Here's how the part is built. I have some questions about the finished solid (model axes, mm). A direction names the side the tool comes from. Coordinates: 2 decimals unless noted, no trailing zeros. Order: outer loops, then holes, each group sorted by start corner. A loop starts at its lowest first (then second) coordinate and runs counter-clockwise, first axis right, second up. Notation, with made-up numbers: (-8, -31) - (6, -31) arc R24 cw to (6, -5) - close; hole circle Ø4 at (-28, 10.5). An arc over 180 degrees is marked (long way). Answer in a Markdown table with one row per item. Add a question column.
Item 1: I want a section at A-A (z = 6). Please give me the cut outline in (x, y).
Item 2: On a 3-axis mill with a long thin cutter (end or side, diameter ignored), from which of +Z, -Z, +X, -X, +Y, -Y can I reach the whole of each face in a straight line? I mean faces 1 (the flat face through (44.45, 23, 27)), 2 (the cylindrical face through (15.755, -35.203, 37.922)), 3 (the flat face through (5.08, 32, 39)), 4 (the flat face through (7, -25.4, 7)). Say none if no direction works.
Item 3: I want a section at B-B (x = 9.5). Please give me the cut outline in (y, z).
Item 4: Will these pins go through, and if not, where does the flat tip stop? pin 1 Ø4.5 at (y, z) = (31.5, 42) entering from -X; pin 2 Ø8 at (x, y) = (21, -28.5) entering from +Z.
Item 5: If I drill on line 1 along Y through (x, z) = (37, 39.5); line 2 along Y through (x, z) = (29.5, 45.5); line 3 along Y through (x, z) = (5, 4), over which ranges is the centre line in solid material (lowest first)? Write a range as from..to.
Item 6: I want a section at D-D (z = 44). Please give me the cut outline in (x, y), plus the area to 3 significant figures.
Item 7: I want a section at C-C (y = -2). Please give me the cut outline in (x, z).
```python
from build123d import *

# Parameters (mm, degrees)
F0_W      = 50.8
F0_H      = 50.8
F1_DEPTH  = 50.8
F2_W      = 25.4
F2_H      = 25.4
F3_DEPTH  = 25.4
F4_R      = 10.16
F5_W      = 12.7
F5_H      = 12.7
F6_DEPTH  = 6.35
F7_R      = 5.08
F10_DEPTH = 25.4
F13_R     = 7.816063
F14_DEPTH = 5.08


with BuildPart() as f1:
    # F0 (on Top) → F1 (new body)
    with BuildSketch(Plane.XY):
        with Locations((25.4, 25.4)):
            Rectangle(F0_W, F0_H)
    extrude(amount=F1_DEPTH)

    # F2 (on face) → F3 (cut)
    with BuildSketch(Plane.XY.offset(50.8)):
        with Locations((25.4, 25.4)):
            Rectangle(F2_W, F2_H)
    extrude(amount=-F3_DEPTH, mode=Mode.SUBTRACT)

    # F4
    f4_edges = [f1.edges().sort_by_distance(p)[0] for p in [
        (12.7, 38.1, 38.1),
        (38.1, 38.1, 38.1),
        (12.7, 12.7, 38.1),
        (38.1, 12.7, 38.1),
    ]]
    fillet(f4_edges, radius=F4_R)

    # F5 (on face) → F6 (cut)
    with BuildSketch(Plane.YZ.offset(50.8)):
        with Locations((23.145751, 26.69926)):
            Rectangle(F5_W, F5_H)
    extrude(amount=-F6_DEPTH, mode=Mode.SUBTRACT)

    # F7
    f7_edges = [f1.edges().sort_by_distance(p)[0] for p in [
        (47.625, 16.795751, 20.34926),
        (47.625, 16.795751, 33.04926),
        (47.625, 29.495751, 33.04926),
        (47.625, 29.495751, 20.34926),
    ]]
    fillet(f7_edges, radius=F7_R)

    # F9 (on face) → F10 (cut)
    with BuildSketch(Plane.XZ):
        Polygon((0, 25.4), (0, 0), (25.4, 0), align=None)
    extrude(amount=-F10_DEPTH, mode=Mode.SUBTRACT)

    # F12: F1 across face


with BuildPart() as f1_1:
    add(f1.part)
    add(f1.part.mirror(Plane(origin=(27.819048, 0, 27.819048), x_dir=(1, 0, 0), z_dir=(0, -1, 0))))

    # F13 (on face) → F14 (cut)
    with BuildSketch(Plane(origin=(0, 0, 0), x_dir=(0, -1, 0), z_dir=(-1, 0, 0))):
        with Locations((-31.531367, 39.15615)):
            Circle(F13_R)
    extrude(amount=-F14_DEPTH, mode=Mode.SUBTRACT)


solid = f1_1.part
```
Values follow:
| question | item | result |
|---|---|---|
| 1 | outline | (0, -50.8) - (50.8, -50.8) - (50.8, 50.8) - (0, 50.8) - (0, 25.4) - (19.4, 25.4) - (19.4, -25.4) - (0, -25.4) - close |
| 2 | face 1 | +X |
| 2 | face 2 | +Z |
| 2 | face 3 | -X |
| 2 | face 4 | -Z, -X |
| 3 | outline | (-50.8, 0) - (-25.4, 0) - (-25.4, 15.9) - (25.4, 15.9) - (25.4, 0) - (50.8, 0) - (50.8, 50.8) - (-50.8, 50.8) - close |
| 4 | pin 1 | stops at x = 5.08 |
| 4 | pin 2 | stops at z = 25.4 |
| 5 | line 1 | y = -50.8..-32.54, -18.26..18.26, 32.54..50.8 |
| 5 | line 2 | y = -50.8..-37.98, -12.82..12.82, 37.98..50.8 |
| 5 | line 3 | y = -50.8..-25.4, 25.4..50.8 |
| 6 | outline | (0, -50.8) - (50.8, -50.8) - (50.8, 50.8) - (0, 50.8) - (0, 37.67) - (5.08, 37.67) - (5.08, 25.4) - (0, 25.4) - close; hole (12.7, -27.94) arc R10.16 ccw to (22.86, -38.1) - (27.94, -38.1) arc R10.16 ccw to (38.1, -27.94) - (38.1, -22.86) arc R10.16 ccw to (27.94, -12.7) - (22.86, -12.7) arc R10.16 ccw to (12.7, -22.86) - close; hole (12.7, 22.86) arc R10.16 ccw to (22.86, 12.7) - (27.94, 12.7) arc R10.16 ccw to (38.1, 22.86) - (38.1, 27.94) arc R10.16 ccw to (27.94, 38.1) - (22.86, 38.1) arc R10.16 ccw to (12.7, 27.94) - close |
| 6 | area | 3,990 mm^2 |
| 7 | outline | (0, 25.4) - (25.4, 0) - (50.8, 0) - (50.8, 50.8) - (0, 50.8) - close |
